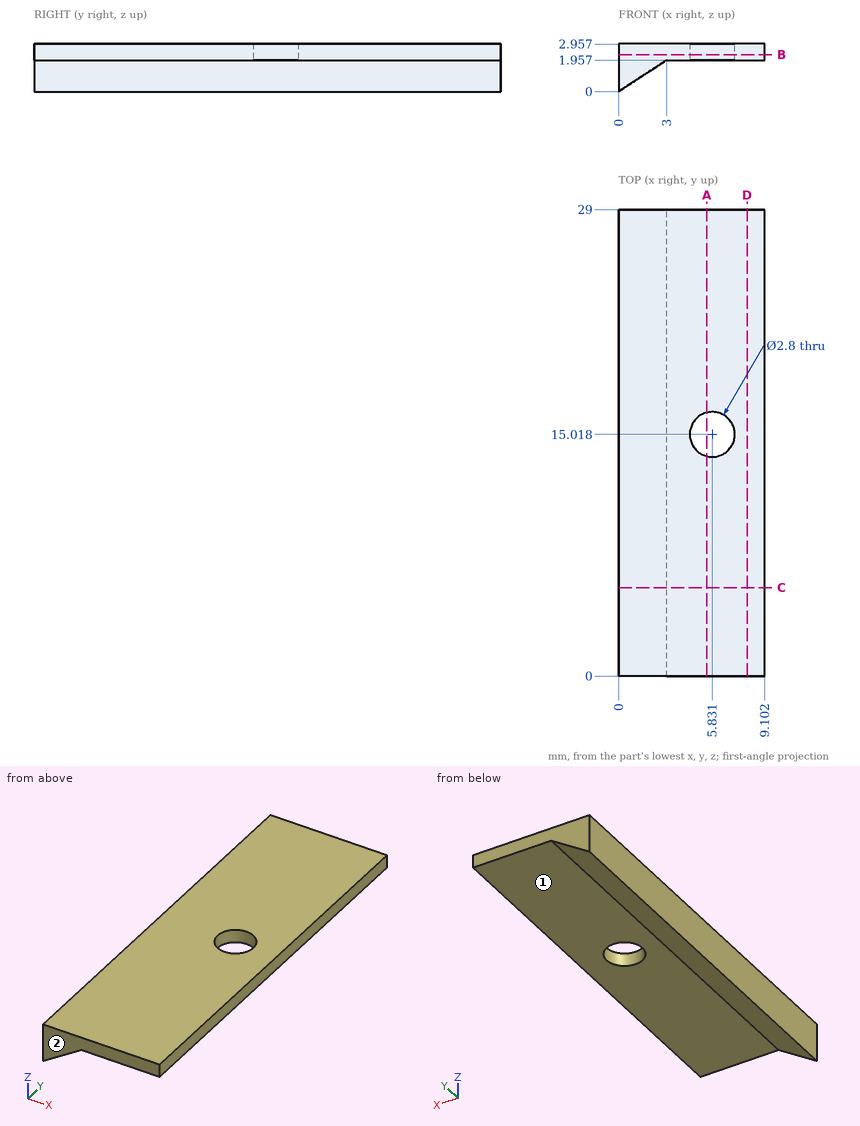
Input: dimensioned drawing with shaded views. Units: mm. Origin: part minimum x, y, z. A direction names the side the tool comes from. Give positions to 0.01 mm unless a question says otherwise; leave off trailing zeros. Write each loop counter-clockwise with the first axis right and the second up, starting at its lowest first coordinate (ties: lowest second). Pieces come first, ordered by that corner, then holes.
1. Section query C-C (y = 5.5). Return the cut outline in (x, z).
2. Material intervals for line 1 along Z through (x, y) = (8.25, 12); line 2 along Y through (x, z) = (6.25, 2.7) (1 decimal); line 3 along Z through (x, y) = (1.25, 19.75) (1 decimal), sorted ascending.
3. Section query B-B (z = 2.3). Return the cut outline in (x, y).
4. Section query D-D (x = 8). Return the cut outline in (y, z), then the cut area to 3 significant figures.
5. Section query A-A (x = 5.5). Return the cut outline in (y, z).
6. Access query for the marked faces 1 and 2. Directions: +Z, -Z, +X, -X, +Y, -Y. A direction counts if a zero-diameter tool reaches every point of the face in a straight line with its end or side. Return the directions, or none.
7. First-contact query: pin 1 (5 mm diameter, centred on x = 5, y = 13.5, fed in from -Z). Flat tip, straight axial feed; report the tip coordinate or a pass-through.
Output values:
1. outline: (0, 0) - (3, 1.96) - (9.1, 1.96) - (9.1, 2.96) - (0, 2.96) - close
2. line 1: z = 1.96 to 2.96
2. line 2: y = 0 to 13.7, 16.4 to 29
2. line 3: z = 0.8 to 3
3. outline: (0, 0) - (9.1, 0) - (9.1, 29) - (0, 29) - close; hole circle Ø2.8 at (5.83, 15.02)
4. outline: (0, 1.96) - (29, 1.96) - (29, 2.96) - (0, 2.96) - close
4. area: 29.0 mm2
5. outline: (0, 1.96) - (13.66, 1.96) - (13.66, 2.96) - (0, 2.96) - close; (16.38, 1.96) - (29, 1.96) - (29, 2.96) - (16.38, 2.96) - close
6. face 1: -Z, +X, +Y, -Y
6. face 2: +Z, -Z, +X, -X, -Y
7. pin 1: stops at z = 1.63
